Autodesk Inventor part; units mm, degrees
ref_plane "YZ Plane" through (0, 0, 0) normal (1, 0, 0) x (0, 1, 0)
ref_plane "XZ Plane" through (0, 0, 0) normal (0, 1, 0) x (-1, 0, 0)
ref_plane "XY Plane" through (0, 0, 0) normal (0, 0, 1) x (1, 0, 0)
sketch "Sketch1" plane through (0, 0, 0) normal (0, 1, 0) x (-1, 0, 0)
  line L0 (46.76465, 19.785927) -> (46.76465, -5.614073)
  line L1 (46.76465, -5.614073) -> (-34.05815, -5.614073)
  line L2 (-34.05815, -5.614073) -> (-34.05815, 19.785927)
  line L3 (-34.05815, 19.785927) -> (46.76465, -5.614073) construction
  line L4 (46.76465, 19.785927) -> (-34.05815, -5.614073) construction
  line L5 (-34.05815, 19.785927) -> (-34.05815, 50.011927)
  line L6 (46.76465, 19.785927) -> (46.76465, 50.011927)
  line L7 (46.76465, 19.785927) -> (-34.05815, 19.785927)
  line L8 (46.76465, 19.785927) -> (6.35325, 19.785927)
  line L9 (46.76465, 50.011927) -> (37.59525, 50.011927)
  line L10 (-23.87275, 50.011927) -> (-34.05815, 50.011927)
  line L11 (37.59525, 50.011927) -> (36.32525, 50.011927)
  arc A0 (-24.12675, 50.011927) -> (36.32525, 50.011927) centre (6.09925, 50.011927) ccw
  point P0 (6.35325, 7.085927)
  dimension "d11" = 80.8228
  dimension "d12" = 25.4
  dimension "d13" = 30.226
  dimension "d14" = 30.226
  dimension "d40" = 40.4114
  dimension "d46" = 60.452
sketch "Sketch1 outline for Extrusion3" plane through (0, 0, 0) normal (0, 1, 0) x (-1, 0, 0)
  line L0 (-34.05815, 50.011927) -> (-34.05815, 19.785927)
  line L1 (-24.12675, 50.011927) -> (-34.05815, 50.011927)
  arc A0 (36.32525, 50.011927) -> (-24.12675, 50.011927) centre (6.09925, 50.011927) cw
  line L2 (37.59525, 50.011927) -> (36.32525, 50.011927)
  line L3 (46.76465, 50.011927) -> (37.59525, 50.011927)
  line L4 (46.76465, 19.785927) -> (46.76465, 50.011927)
  line L5 (46.76465, -5.614073) -> (46.76465, 19.785927)
  line L6 (-34.05815, -5.614073) -> (46.76465, -5.614073)
  line L7 (-34.05815, 19.785927) -> (-34.05815, -5.614073)
extrude "Extrusion3" add sketch "Sketch1 outline for Extrusion3" along normal blind 1.5875
sketch "Sketch2" plane through (0, 1.5875, 0) normal (0, 1, 0) x (1, 0, 0)
  line L0 (34.05815, 5.614073) -> (-46.76465, 5.614073)
  line L1 (34.05815, 5.614073) -> (34.05815, -19.785927)
  line L2 (34.05815, -50.011927) -> (34.05815, 5.614073)
  line L3 (34.05815, 5.614073) -> (34.05815, -0.735927)
  line L4 (34.05815, -0.735927) -> (19.04675, -0.735927)
  circle A0 centre (19.04675, -0.735927) radius 2.1844
  line L5 (34.05815, 5.614073) -> (34.05815, -7.085927)
  line L6 (34.05815, -7.085927) -> (-0.00325, -7.085927)
  circle A1 centre (-0.00325, -7.085927) radius 2.1844
  line L7 (19.04675, -0.735927) -> (-31.75325, -0.735927)
  circle A2 centre (-31.75325, -0.735927) radius 2.1844
  arc A3 (-46.76465, -56.057127) -> (-44.93585, -57.885927) centre (-44.93585, -56.057127) ccw
  arc A4 (32.22935, -57.885927) -> (34.05815, -56.057127) centre (32.22935, -56.057127) ccw
  line L8 (34.05815, -19.785927) -> (-46.76465, -19.785927)
  line L9 (-46.76465, 5.614073) -> (-46.76465, -50.011927)
  line L10 (34.05815, -19.785927) -> (34.05815, -24.865927)
  line L11 (34.05815, -24.865927) -> (21.99315, -24.865927)
  circle A5 centre (21.99315, -24.865927) radius 2.1844
  line L12 (-46.76465, -19.785927) -> (-46.76465, -24.865927)
  line L13 (-46.76465, -24.865927) -> (-34.69965, -24.865927)
  circle A6 centre (-34.69965, -24.865927) radius 2.1844
  point P0 (0, 0)
  point P1 (-31.057127, -40.306856)
  point P2 (31.050628, -40.30613)
  point P3 (-43.267434, -44.121852)
  point P4 (30.560934, -44.122114)
  dimension "d18" = 25.4
  dimension "d19" = 6.35
  dimension "d20" = 15.0114
  dimension "d21" = 4.3688
  dimension "d22" = 12.7
  dimension "d23" = 34.0614
  dimension "d24" = 4.3688
  dimension "d25" = 50.8
  dimension "d26" = 4.3688
  dimension "d30" = 5.08
  dimension "d31" = 12.065
  dimension "d32" = 4.3688
  dimension "d33" = 5.08
  dimension "d34" = 12.065
  dimension "d35" = 4.3688
extrude "Extrusion4" cut sketch "Sketch2" against normal blind 1.5875 contours A0 L7 L4 | L4 L7 A0 | A1 | A2 | A5 | A6
fillet "Fillet2" radius 3.175 4 edges at (-46.7646, 0.7937, 50.0119) (34.0582, 0.7937, 50.0119) (-36.3252, 0.7937, 50.0119) (24.1268, 0.7937, 50.0119)
equation "\"d31\" = d34"
equation "\"BendRadius\" = Thickness"
equation "\"BendReliefWidth\" = Thickness"
equation "\"BendReliefDepth\" = 0.5 * Thickness"
equation "\"CornerReliefSize\" = 4 * Thickness"
equation "\"MinimumRemnant\" = 2 * Thickness"
equation "\"TransitionRadius\" = BendRadius"
equation "\"JacobiRadiusSize\" = BendRadius"
equation "\"GapSize\" = Thickness"
properties part number "Winter-Climb-Guides" material "Polycarbonate, Clear"
Check sheet for the modelled part. Datum: model origin and axes. Units: mm. A direction names the side the tool comes from. Give positions to 0.01 mm unless a question says otherwise; leave off trailing zeros. Write each loop counter-clockwise with the first axis right and the second up, starting at its lowest first coordinate (ties: lowest second). Pieces come first, ordered by that corner, then holes. Notation, with made-up numbers: (6, 35.25) -> (58, 35.25) arc R24 cw to (58, 62.25) -> close; hole circle Ø10 at (-2.75, 19.25). An arc over 180 degrees is marked (long way). Use one line per item in the form item = value. Start each with the question number.
1. Section check A-A (z = 28.5). Record the cut outline in (x, y), and give its area (3 significant figures).
2. Mould release check, pull along X, two halves, no side actions. Record for faces 3 (the flat face through (-6, 1, -5.614)), 4 (the cylindrical face through (-37.24, 0.8, 49.21)), 5 (the cylindrical face through (33.1, 0.8, 49.11)): pulls with the +X half, pulls with the -X half, needs draft (parallel to the pull), parting line crosses it, or undercut.
3. Section check D-D (x = 11.5). Record the cut outline in (y, z), and give its area (3 significant figures).
4. Section check B-B (y = 0.9). Count the separate pieces of the cut face and the enclosed holes in it, and give its area (3 significant figures).
5. Section check C-C (x = 22.5). Record the cut outline in (y, z).
6. Access from +Z, -Z, +X, -X, +Y, -Y to the whole of each face (thin tool, end or side, straight path). Record for faces 1 (the cylindrical face through (24.991, 0.805, 49.164)), 2 (the cylindrical face through (17.313, 0.805, 2.065)).
7. Thickness scan on line 1 along X through (y, z) = (0.45, 23); line 2 along X through (y, z) = (0.65, 0); line 3 along X through (y, z) = (0.45, 30.5). Record the ranges inside material, lowest first. Write a range as from..to.
Conclusion:
q1.outline = (-46.76, 0) -> (-27.33, 0) -> (-27.33, 1.59) -> (-46.76, 1.59) -> close; (15.13, 0) -> (34.06, 0) -> (34.06, 1.59) -> (15.13, 1.59) -> close
q1.area = 60.9 mm²
q2.face_3 = needs draft
q2.face_4 = undercut
q2.face_5 = pulls with the +X half
q3.outline = (0, -5.61) -> (1.59, -5.61) -> (1.59, 25.44) -> (0, 25.44) -> close
q3.area = 49.3 mm²
q4.separate_pieces = 1
q4.enclosed_holes = 5
q4.area = 2,980 mm²
q5.outline = (0, -5.61) -> (1.59, -5.61) -> (1.59, 22.74) -> (0, 22.74) -> close; (0, 26.99) -> (1.59, 26.99) -> (1.59, 40.23) -> (0, 40.23) -> close
q6.face_1 = +Z, +Y, -Y
q6.face_2 = +Y, -Y
q7.line_1 = -46.76..-35.84, -33.56..-19.66, 7.46..20.86, 23.13..34.06
q7.line_2 = -46.76..-33.81, -29.7..16.99, 21.1..34.06
q7.line_3 = -46.76..-29.18, 16.99..34.06
